Geometry: final body of the model. Coordinates: model frame, mm. A direction names the side the tool comes from. Coordinates: 2 decimals unless noted, no trailing zeros. Order: outer loops, then holes, each group sorted by start corner. A loop starts at its lowest first (then second) coordinate and runs counter-clockwise, first axis right, second up. Notation, with made-up numbers: M -38,7 L -7,7 A25 cw -7,26 Z; hole C 9,33.25 d2. An arc over 180 degrees is marked long. Write item = value, one per line.
from build123d import *

# Parameters (mm, degrees)
SKETCH1_R               = 39
BOSS_EXTRUDE1_DEPTH     = 321
SKETCH2_OUTSIDE_W       = 147.884
SKETCH2_OUTSIDE_H       = 147.884
SKETCH2_OUTSIDE_R       = 25
CUT_EXTRUDE1_DEPTH      = 250
SKETCH3_OUTSIDE_W       = 147.884
SKETCH3_OUTSIDE_H       = 147.884
SKETCH3_OUTSIDE_R       = 22
CUT_EXTRUDE2_DEPTH      = 28
SKETCH4_R               = 13
CUT_EXTRUDE3_DEPTH      = 91
CUT_EXTRUDE4_DEPTH      = 326.703853216
CUT_EXTRUDE4_DEPTH_BACK = 25
CUT_EXTRUDE5_DEPTH      = 326.703853216
CUT_EXTRUDE5_DEPTH_BACK = 25
SKETCH7_OUTSIDE_W       = 147.884
SKETCH7_OUTSIDE_H       = 147.884
SKETCH7_OUTSIDE_R       = 12.5
CUT_EXTRUDE6_DEPTH      = 70
CUT_EXTRUDE7_DEPTH      = 326.703853216
CUT_EXTRUDE7_DEPTH_BACK = 10
CUT_EXTRUDE8_DEPTH      = 326.703853216
CUT_EXTRUDE8_DEPTH_BACK = 10
SKETCH10_R              = 6
CUT_EXTRUDE9_DEPTH      = 326.703853216


with BuildPart() as part:
    # Sketch1 → Boss-Extrude1 (new body)
    with BuildSketch(Plane.XY):
        Circle(SKETCH1_R)
    extrude(amount=BOSS_EXTRUDE1_DEPTH)

    # Sketch2 outside → Cut-Extrude1 (cut)
    with BuildSketch(Plane.XY.offset(321)):
        Rectangle(SKETCH2_OUTSIDE_W, SKETCH2_OUTSIDE_H)
        Circle(SKETCH2_OUTSIDE_R, mode=Mode.SUBTRACT)
    extrude(amount=-CUT_EXTRUDE1_DEPTH, mode=Mode.SUBTRACT)

    # Sketch3 outside → Cut-Extrude2 (cut)
    with BuildSketch(Plane(origin=(0, 0, 0), x_dir=(-1, 0, 0), z_dir=(0, 0, -1))):
        Rectangle(SKETCH3_OUTSIDE_W, SKETCH3_OUTSIDE_H)
        Circle(SKETCH3_OUTSIDE_R, mode=Mode.SUBTRACT)
    extrude(amount=-CUT_EXTRUDE2_DEPTH, mode=Mode.SUBTRACT)

    # Sketch4 → Cut-Extrude3 (cut)
    with BuildSketch(Plane(origin=(0, 0, 0), x_dir=(-1, 0, 0), z_dir=(0, 0, -1))):
        Circle(SKETCH4_R)
    extrude(amount=-CUT_EXTRUDE3_DEPTH, mode=Mode.SUBTRACT)

    # Sketch5 → Cut-Extrude4 (cut, two sides: drawn at the far end of the back side and taken through both)
    with BuildSketch(Plane(origin=(0, 0, 0), x_dir=(-1, 0, 0), z_dir=(0, 0, -1)).offset(-CUT_EXTRUDE4_DEPTH_BACK)):
        Polygon((179.395153858, -16), (15.099668871, -16), (-15.099668871, -16), (-179.395153858, -16), (-179.395153858, -344.590969976), (179.395153858, -344.590969976), align=None)
    extrude(amount=CUT_EXTRUDE4_DEPTH + CUT_EXTRUDE4_DEPTH_BACK, mode=Mode.SUBTRACT)

    # Sketch6 → Cut-Extrude5 (cut, two sides: drawn at the far end of the back side and taken through both)
    with BuildSketch(Plane(origin=(0, 0, 0), x_dir=(-1, 0, 0), z_dir=(0, 0, -1)).offset(-CUT_EXTRUDE5_DEPTH_BACK)):
        Polygon((179.395153858, 16), (15.099668871, 16), (-15.099668871, 16), (-179.395153858, 16), (-179.395153858, 344.590969976), (179.395153858, 344.590969976), align=None)
    extrude(amount=CUT_EXTRUDE5_DEPTH + CUT_EXTRUDE5_DEPTH_BACK, mode=Mode.SUBTRACT)

    # Sketch7 outside → Cut-Extrude6 (cut)
    with BuildSketch(Plane.XY.offset(321)):
        Rectangle(SKETCH7_OUTSIDE_W, SKETCH7_OUTSIDE_H)
        Circle(SKETCH7_OUTSIDE_R, mode=Mode.SUBTRACT)
    extrude(amount=-CUT_EXTRUDE6_DEPTH, mode=Mode.SUBTRACT)

    # Sketch8 → Cut-Extrude7 (cut, two sides: drawn at the far end of the back side and taken through both)
    with BuildSketch(Plane.XY.offset(321).offset(-CUT_EXTRUDE7_DEPTH_BACK)):
        Polygon((-154.459376077, 8.5), (-9.16515139, 8.5), (9.16515139, 8.5), (154.459376077, 8.5), (154.459376077, 299.088449374), (-154.459376077, 299.088449374), align=None)
    extrude(amount=CUT_EXTRUDE7_DEPTH + CUT_EXTRUDE7_DEPTH_BACK, mode=Mode.SUBTRACT)

    # Sketch9 → Cut-Extrude8 (cut, two sides: drawn at the far end of the back side and taken through both)
    with BuildSketch(Plane.XY.offset(321).offset(-CUT_EXTRUDE8_DEPTH_BACK)):
        Polygon((-154.459376077, -8.5), (-9.16515139, -8.5), (9.16515139, -8.5), (154.459376077, -8.5), (154.459376077, -299.088449374), (-154.459376077, -299.088449374), align=None)
    extrude(amount=CUT_EXTRUDE8_DEPTH + CUT_EXTRUDE8_DEPTH_BACK, mode=Mode.SUBTRACT)

    # Sketch10 → Cut-Extrude9 (cut, through all)
    with BuildSketch(Plane.XY.offset(321)):
        Circle(SKETCH10_R)
    extrude(amount=-CUT_EXTRUDE9_DEPTH, mode=Mode.SUBTRACT)


solid = part.part
1) Set-up query: faces 4 (the face through (0, -16, 13)), 5 (the face through (-12.488, 0.55, 286.49)), 6 (the face through (0, -8.5, 316)). Return all of +Z, -Z, +X, -X, +Y, -Y with unobstructed straight access to the full face (end or side cutting, diameter ignored); none if empty.
Numbers:
face_4 = -Z, +X, -X, -Y
face_5 = +Z
face_6 = +Z, +X, -X, -Y
2) Section A-A, the plane y = 0. Return loops of the section in (x, z).
Numbers:
outline = M -39,28 L -22,28 L -22,0 L -13,0 L -13,91 L -6,91 L -6,321 L -12.5,321 L -12.5,251 L -25,251 L -25,71 L -39,71 Z; M 6,91 L 13,91 L 13,0 L 22,0 L 22,28 L 39,28 L 39,71 L 25,71 L 25,251 L 12.5,251 L 12.5,321 L 6,321 Z
3) Section C-C, the plane z = 65. Return loops of the section in (x, y).
Numbers:
outline = C 0,0 d78; hole C 0,0 d26
4) Mould query, pull axis X, two halves, no side actions, for faces 1 (the face through (-6, -3, 91)), 2 (the face through (0, 8.5, 316)), 3 (the face through (23.846, 7.509, 162.26)). Classes: pulls with the +X half, pulls with the -X half, needs draft (parallel to the pull), parting line crosses it, or undercut.
Numbers:
face_1 = undercut
face_2 = needs draft
face_3 = parting line crosses it
5) Section D-D, the plane z = 138. Return loops of the section in (x, y), and give its area (3 significant figures).
Numbers:
outline = C 0,0 d50; hole C 0,0 d12
area = 1,850 mm²
6) Pin query (flat end, axial travel): pin 1 (5 mm diameter, centred on x = 3.5, z = 314, fed in from +Y); pin 2 (3 mm diameter, centred on x = 6, y = -19.5, fed in from -Z); pin 3 (20 mm diameter, centred on x = 2.5, z = 17, fed in from +Y); pin 4 (23.5 mm diameter, centred on x = -8.5, y = -16.5, fed in from -Z). Return the tip coordinate at first contact, or that it passes through.
Numbers:
pin_1 = 8.5
pin_2 = 25
pin_3 = 22
pin_4 = 0
7) Line query: L1, parallel to Y at x = 0, z = 209; L2, parallel to Y at x = 0, z = 258; L3, parallel to Z at x = 8, y = -31.5. Output: solid intervals per line, ascending.
Numbers:
L1 = -25 to -6, 6 to 25
L2 = -12.5 to -6, 6 to 12.5
L3 = 28 to 71
